Geometry check sheet. Reference: drawing and pictorial views, mm from the part's lowest x, y, z. Round coordinates to 2 decimals unless told otherwise and drop trailing zeros. Order: outer loops, then holes, each group sorted by start corner. A loop starts at its lowest first (then second) coordinate and runs counter-clockwise, first axis right, second up. Notation, with made-up numbers: (-18, 42.25) -> (41, 42.25) arc R19 cw to (41, 58.25) -> close; hole circle Ø2 at (37, 62). An arc over 180 degrees is marked (long way). Put each result on its own line as item: value.
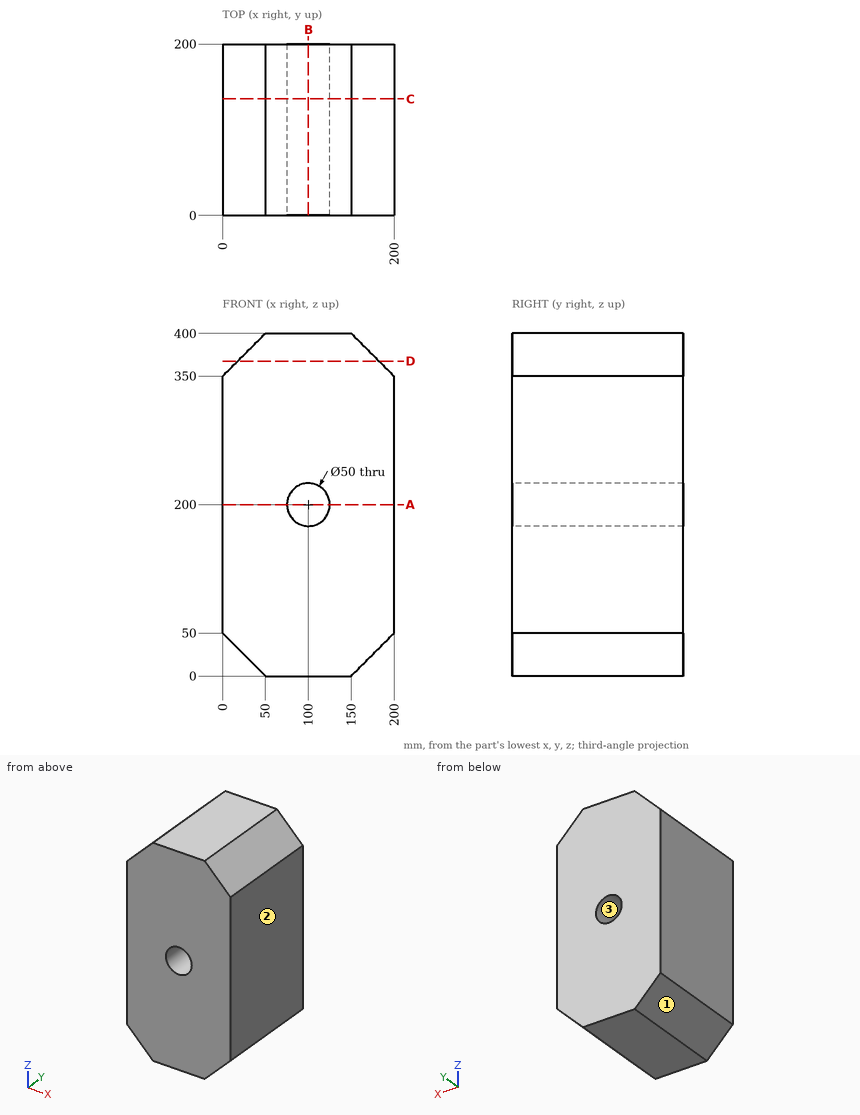
Item 1: Sectioned sample at A-A, the plane z = 200. Record the boundary of the cut face in (x, y), then the cut area to 3 significant figures.
Geometry check:
outline: (0, 0) -> (75, 0) -> (75, 200) -> (0, 200) -> close; (125, 0) -> (200, 0) -> (200, 200) -> (125, 200) -> close
area: 30,000 mm2
Item 2: Release check for a two-part mould opening along X. For the marked faces 1, 2 and 3 record: pulls with the +X half, pulls with the -X half, needs draft (parallel to the pull), parting line crosses it, or undercut.
Geometry check:
face 1: pulls with the -X half
face 2: pulls with the +X half
face 3: undercut
Item 3: Sectioned sample at C-C, the plane y = 136. Record the boundary of the cut face in (x, z).
Geometry check:
outline: (0, 50) -> (50, 0) -> (150, 0) -> (200, 50) -> (200, 350) -> (150, 400) -> (50, 400) -> (0, 350) -> close; hole circle Ø50 at (100, 200)
Item 4: Depth check by flat-ended pin: pin 1 Ø1.5 at (x, y) = (167.5, 24) entering from +Z. Enter the tip coordinate at first touch or a pass-through.
Geometry check:
pin 1: z = 383.25
Item 5: Sectioned sample at D-D, the plane z = 367.5. Record the boundary of the cut face in (x, y), then the cut area to 3 significant figures.
Geometry check:
outline: (17.5, 0) -> (182.5, 0) -> (182.5, 200) -> (17.5, 200) -> close
area: 33,000 mm2
Item 6: Sectioned sample at B-B, the plane x = 100. Record the boundary of the cut face in (y, z), then the cut area to 3 significant figures.
Geometry check:
outline: (0, 0) -> (200, 0) -> (200, 175) -> (0, 175) -> close; (0, 225) -> (200, 225) -> (200, 400) -> (0, 400) -> close
area: 70,000 mm2
Item 7: Material ranges on line 1 along Z through (x, y) = (100, 144); line 2 along X through (y, z) = (192, 204); line 3 along Z through (x, y) = (107.5, 85.5), recorded low to high.
Geometry check:
line 1: 0 to 175, 225 to 400
line 2: 0 to 75.32, 124.68 to 200
line 3: 0 to 176.15, 223.85 to 400
